Could you check a few things on this model? Use its own coordinates, in mm. A direction names the side the tool comes from. Round coordinates to 2 decimals unless told otherwise and drop trailing zeros. Order: outer loops, then holes, each group sorted by start corner. A loop starts at its lowest first (then second) coordinate and runs counter-clockwise, first axis right, second up. Notation, with made-up numbers: (32.25, -5.5) - (52.25, -5.5) arc R11 cw to (52.25, 2.5) - close; hole circle Ø10 at (89, 40.25). An arc over 180 degrees is marked (long way). Use one line per item in the form item = value.
from build123d import *

# Parameters (mm, degrees)
ESTRUSIONE_ESTRUSIONE1_DEPTH = 20
M4_CLEARANCE_HOLE1_D         = 4.5
RACCORDO1_R                  = 5
SCHIZZO4_W                   = 9
SCHIZZO4_H                   = 2.5
SCHIZZO4_W_2                 = 8.5
ESTRUSIONE_ESTRUSIONE2_DEPTH = 1.5


with BuildPart() as part:
    # Schizzo1 → Estrusione-Estrusione1 (new body)
    with BuildSketch(Plane.XY):
        Polygon((0, 30.6), (-5, 30.6), (-5, 20.1), (-10.5, 20.1), (-10.5, -5), (-5, -5), (-5, -15.5), (0, -15.5), (0, 0), (-5.5, 0), (-5.5, 15.1), (0, 15.1), align=None)
    extrude(amount=ESTRUSIONE_ESTRUSIONE1_DEPTH)

    # M4 Clearance Hole1 (through all)
    with Locations(Plane.ZY.offset(5)):
        with Locations((10, 24.6), (10, -9.5)):
            Hole(M4_CLEARANCE_HOLE1_D / 2)

    # Raccordo1
    raccordo1_edges = [part.edges().sort_by_distance(p)[0] for p in [
        (-10.5, -5, 10),
        (-10.5, 20.1, 10),
    ]]
    fillet(raccordo1_edges, radius=RACCORDO1_R)

    # Schizzo4 → Estrusione-Estrusione2 (add)
    with BuildSketch(Plane(origin=(-5.5, 0, 0), x_dir=(0, 0, -1), z_dir=(1, 0, 0))):
        with Locations((-15.5, 6.85)):
            Rectangle(SCHIZZO4_W, SCHIZZO4_H)
        with Locations((-4.25, 6.85)):
            Rectangle(SCHIZZO4_W_2, SCHIZZO4_H)
    extrude(amount=ESTRUSIONE_ESTRUSIONE2_DEPTH)


solid = part.part
Item 1: I need wall thicknesses on L1, parallel to Y at x = -3.9, z = 10; L2, parallel to Y at x = -2.25, z = 12; L3, parallel to Y at x = -2, z = 15.25. Which ranges of each line are inside material? Lowest first, please.
Found:
L1 = -15.5 to -11.75, -7.25 to 0, 15.1 to 22.35, 26.85 to 30.6
L2 = -15.5 to -10.53, -8.47 to 0, 15.1 to 23.57, 25.63 to 30.6
L3 = -15.5 to 0, 15.1 to 30.6
Item 2: Will these pins go through, and if not, where does the flat tip stop? P1, Ø2, axis at y = 6.5, z = 14.5, coming from the +X side; P2, Ø0.6, axis at x = -5.5, z = 9, coming from the +Y side; P3, Ø3.5, axis at y = 24.6, z = 10, coming from the +X side; P4, Ø7, axis at y = -9.5, z = 10, coming from the -X side.
Found:
P1 = -4
P2 = 20.1
P3 = through
P4 = -5
Item 3: Imagine slicing it at A-A on x = -2.5. Please give me the cut outline in (y, z).
Found:
outline = (-15.5, 0) - (0, 0) - (0, 20) - (-15.5, 20) - close; (15.1, 0) - (30.6, 0) - (30.6, 20) - (15.1, 20) - close; hole circle Ø4.5 at (-9.5, 10); hole circle Ø4.5 at (24.6, 10)
Item 4: Imagine slicing it at D-D on y = 7.5. Please give me the cut outline in (x, z).
Found:
outline = (-10.5, 0) - (-4, 0) - (-4, 8.5) - (-5.5, 8.5) - (-5.5, 11) - (-4, 11) - (-4, 20) - (-10.5, 20) - close
Item 5: If we mould it in two halves opening along Z, with no side actions, what happens to faces 4 (the face through (-2.47, 26.83, 10.29)), 5 (the face through (-5.3, 7.9, 0)), 6 (the face through (0, -6, 10))? For each: released by +Z, released by -Z, zero draft, split by the parting line, or undercut.
Found:
face_4 = undercut
face_5 = released by -Z
face_6 = zero draft
Item 6: Imagine slicing it at C-C on z = 10. Please give me the cut outline in (x, y), plus the area to 3 significant figures.
Found:
outline = (-10.5, 0) arc R5 ccw to (-5.5, -5) - (-5, -5) - (-5, -7.25) - (0, -7.25) - (0, 0) - (-5.5, 0) - (-5.5, 15.1) - (0, 15.1) - (0, 22.35) - (-5, 22.35) - (-5, 20.1) - (-5.5, 20.1) arc R5 ccw to (-10.5, 15.1) - close; (-5, -15.5) - (0, -15.5) - (0, -11.75) - (-5, -11.75) - close; (-5, 26.85) - (0, 26.85) - (0, 30.6) - (-5, 30.6) - close
area = 230 mm2
Item 7: Imagine slicing it at B-B on y = 24.6. Please give me the cut outline in (x, z), plus the area to 3 significant figures.
Found:
outline = (-5, 0) - (0, 0) - (0, 7.75) - (-5, 7.75) - close; (-5, 12.25) - (0, 12.25) - (0, 20) - (-5, 20) - close
area = 77.5 mm2
Item 8: For faces 1 (the face through (-5, 25.4, 7.6)), 2 (the face through (-3, 0, 10)), 3 (the face through (-5, -10.2, 7.6)), which set-ups out of +Z, -Z, +X, -X, +Y, -Y let a thin tool reach every point of the face, with its end or its side?
Found:
face_1 = +Z, -Z, -X, +Y
face_2 = +Z, -Z, +X
face_3 = +Z, -Z, -X, -Y
